Part model, mm, in its own coordinate system. A direction names the side the tool comes from. Coordinates: 2 decimals unless noted, no trailing zeros. Write each loop counter-clockwise with the first axis right and the second up, starting at its lowest first coordinate (ties: lowest second). Pieces come first, ordered by that corner, then holes. Notation, with made-up numbers: (87.25, 56.25) - (126.25, 56.25) arc R23 cw to (126.25, 93.25) - close; hole circle Ø1 at (-10.5, 48.5). An arc over 180 degrees is marked (long way). Use a Markdown table: item, result.
```python
from build123d import *

# Parameters (mm, degrees)
F1_DEPTH = 15
F2_W     = 390
F2_H     = 15
F3_DEPTH = 190
F4_R     = 50


with BuildPart() as f1:
    # F0 (on Top) → F1 (new body)
    with BuildSketch(Plane.XY):
        with BuildLine():
            Line((-195, 120), (-195, -150))
            Line((-195, -150), (195, -150))
            Line((195, -150), (195, 120))
            ThreePointArc((195, 120), (186.213203, 141.213203), (165, 150))
            Line((165, 150), (-165, 150))
            ThreePointArc((-165, 150), (-186.213203, 141.213203), (-195, 120))
        make_face()
    extrude(amount=F1_DEPTH)

    # F2 (on face) → F3 (join)
    with BuildSketch(Plane.XY.offset(15)):
        with Locations((0, -142.5)):
            Rectangle(F2_W, F2_H)
    extrude(amount=F3_DEPTH)

    # F4
    f4_edges = [f1.edges().sort_by_distance(p)[0] for p in [
        (195, -142.5, 205),
        (-195, -142.5, 205),
    ]]
    fillet(f4_edges, radius=F4_R)


solid = f1.part
```
Item 1: Drill centre lines: probe 1 along Z at (x, y) = (-93.5, -117); probe 2 along Y at (x, z) = (-10, 185.5); probe 3 along Y at (x, z) = (175, 14.5). Where is each one in solid material? Low to high.
From the geometry:
| item | result |
|---|---|
| probe 1 | 0 to 15 |
| probe 2 | -150 to -135 |
| probe 3 | -150 to 148.28 |
Item 2: Which spindle directions (+Z, -Z, +X, -X, +Y, -Y) get a long thin tool onto all of the face, cutting with end or side? Do faces 1 (the face through (-3, 9, 15)), 2 (the face through (186.445, 140.979, 7.395)). Say none if no direction does.
From the geometry:
| item | result |
|---|---|
| face 1 | +Z, +X, -X, +Y |
| face 2 | +Z, -Z, +X, +Y |
Item 3: Band-saw the part on B-B, the plane z = 146.5. Give the cut face in (x, y), then the cut area to 3 significant figures.
From the geometry:
| item | result |
|---|---|
| outline | (-195, -150) - (195, -150) - (195, -135) - (-195, -135) - close |
| area | 5,850 mm^2 |
Item 4: Band-saw the part on A-A, the plane x = -121. Give the cut face in (y, z).
From the geometry:
| item | result |
|---|---|
| outline | (-150, 0) - (150, 0) - (150, 15) - (-135, 15) - (-135, 205) - (-150, 205) - close |
Item 5: Band-saw the part on C-C, the plane y = 72. Give the cut face in (x, z).
From the geometry:
| item | result |
|---|---|
| outline | (-195, 0) - (195, 0) - (195, 15) - (-195, 15) - close |
Item 6: Drop a flat-ended pin along its axis: P1, Ø4, axis at x = 98, z = 94.5, coming from the +Y side. Give the stop position or say it passes through.
From the geometry:
| item | result |
|---|---|
| P1 | y = -135 |
